```python
from build123d import *

# Parameters (mm, degrees)
BOSS_EXTRUDE1_DEPTH = 6.35
CHAMFER1_SIZE       = 5
CHAMFER1_SIZE_2     = 7.672581673
SKETCH2_R           = 5.25
CUT_EXTRUDE1_DEPTH  = 329.158989668
SKETCH3_R           = 11
CUT_EXTRUDE2_DEPTH  = 329.158989668
SKETCH4_R           = 13
CUT_EXTRUDE3_DEPTH  = 329.158989668


with BuildPart() as part:
    # Sketch1 → Boss-Extrude1 (new body)
    with BuildSketch(Plane.XY):
        with BuildLine():
            Line((-221.187703094, 70), (221.187703094, 70))
            ThreePointArc((221.187703094, 70), (0, -232), (-221.187703094, 70))
        make_face()
    extrude(amount=BOSS_EXTRUDE1_DEPTH)

    # Chamfer1
    # the kernel refuses this chamfer: 7.672581673, 5 mm, written as the material it takes off along each edge
    with BuildSketch(Plane(origin=(-221.187703094, 70, -19.287514673), x_dir=(1, 0, 0), z_dir=(0, 0, 1))) as chamfer1_piece_1:
        with BuildLine():
            Line((CHAMFER1_SIZE, 0), (-2.131765618, -7.131765618))
            ThreePointArc((-2.131765618, -7.131765618), (-1.133115382, -3.68670064), (0, 0))
            Line((0, 0), (CHAMFER1_SIZE, 0))
        make_face()
    extrude(amount=44.925029345, mode=Mode.SUBTRACT)
    with BuildSketch(Plane(origin=(221.187703094, 70, -19.865544851), x_dir=(-1, 0, 0), z_dir=(0, 0, 1))) as chamfer1_piece_2:
        with BuildLine():
            Line((CHAMFER1_SIZE_2, 0), (-1.44240767, 4.732597867))
            ThreePointArc((-1.44240767, 4.732597867), (-0.765078162, 2.465098705), (0, 0))
            Line((0, 0), (CHAMFER1_SIZE_2, 0))
        make_face()
    extrude(amount=46.081089702, mode=Mode.SUBTRACT)

    # Sketch2 → Cut-Extrude1 (cut, through all)
    with BuildSketch(Plane.XY.offset(6.35)):
        with Locations((-190, 0)):
            Circle(SKETCH2_R)
        with Locations((190, 0)):
            Circle(SKETCH2_R)
        with Locations((95, -164.544826719)):
            Circle(SKETCH2_R)
        with Locations((-95, -164.544826719)):
            Circle(SKETCH2_R)
    extrude(amount=-CUT_EXTRUDE1_DEPTH, mode=Mode.SUBTRACT)

    # Sketch3 → Cut-Extrude2 (cut, through all)
    with BuildSketch(Plane.XY.offset(6.35)):
        with Locations((12.5, -30)):
            Circle(SKETCH3_R)
        with Locations((12.5, -55)):
            Circle(SKETCH3_R)
        with Locations((12.5, -80)):
            Circle(SKETCH3_R)
        with Locations((12.5, -105)):
            Circle(SKETCH3_R)
        with Locations((37.5, -30)):
            Circle(SKETCH3_R)
        with Locations((37.5, -55)):
            Circle(SKETCH3_R)
        with Locations((62.5, -30)):
            Circle(SKETCH3_R)
        with Locations((62.5, -55)):
            Circle(SKETCH3_R)
        with Locations((87.5, -30)):
            Circle(SKETCH3_R)
        with Locations((87.5, -55)):
            Circle(SKETCH3_R)
        with Locations((112.5, -30)):
            Circle(SKETCH3_R)
        with Locations((112.5, -55)):
            Circle(SKETCH3_R)
        with Locations((137.5, -30)):
            Circle(SKETCH3_R)
        with Locations((137.5, -55)):
            Circle(SKETCH3_R)
        with Locations((162.5, -30)):
            Circle(SKETCH3_R)
        with Locations((162.5, -55)):
            Circle(SKETCH3_R)
        with Locations((187.5, -30)):
            Circle(SKETCH3_R)
        with Locations((187.5, -55)):
            Circle(SKETCH3_R)
        with Locations((212.5, -30)):
            Circle(SKETCH3_R)
        with Locations((212.5, -55)):
            Circle(SKETCH3_R)
        with Locations((37.5, -80)):
            Circle(SKETCH3_R)
        with Locations((37.5, -105)):
            Circle(SKETCH3_R)
        with Locations((62.5, -80)):
            Circle(SKETCH3_R)
        with Locations((62.5, -105)):
            Circle(SKETCH3_R)
        with Locations((87.5, -80)):
            Circle(SKETCH3_R)
        with Locations((87.5, -105)):
            Circle(SKETCH3_R)
        with Locations((112.5, -80)):
            Circle(SKETCH3_R)
        with Locations((112.5, -105)):
            Circle(SKETCH3_R)
        with Locations((137.5, -80)):
            Circle(SKETCH3_R)
        with Locations((137.5, -105)):
            Circle(SKETCH3_R)
        with Locations((162.5, -80)):
            Circle(SKETCH3_R)
        with Locations((162.5, -105)):
            Circle(SKETCH3_R)
        with Locations((187.5, -80)):
            Circle(SKETCH3_R)
        with Locations((187.5, -105)):
            Circle(SKETCH3_R)
        with Locations((12.5, 30)):
            Circle(SKETCH3_R)
        with Locations((12.5, 55)):
            Circle(SKETCH3_R)
        with Locations((37.5, 55)):
            Circle(SKETCH3_R)
        with Locations((37.5, 30)):
            Circle(SKETCH3_R)
        with Locations((62.5, 55)):
            Circle(SKETCH3_R)
        with Locations((62.5, 30)):
            Circle(SKETCH3_R)
        with Locations((87.5, 55)):
            Circle(SKETCH3_R)
        with Locations((87.5, 30)):
            Circle(SKETCH3_R)
        with Locations((112.5, 55)):
            Circle(SKETCH3_R)
        with Locations((112.5, 30)):
            Circle(SKETCH3_R)
        with Locations((137.5, 55)):
            Circle(SKETCH3_R)
        with Locations((137.5, 30)):
            Circle(SKETCH3_R)
        with Locations((162.5, 55)):
            Circle(SKETCH3_R)
        with Locations((162.5, 30)):
            Circle(SKETCH3_R)
        with Locations((187.5, 55)):
            Circle(SKETCH3_R)
        with Locations((187.5, 30)):
            Circle(SKETCH3_R)
        with Locations((212.5, 55)):
            Circle(SKETCH3_R)
        with Locations((212.5, 30)):
            Circle(SKETCH3_R)
    cut_extrude2 = extrude(amount=-CUT_EXTRUDE2_DEPTH, mode=Mode.SUBTRACT)

    # Mirror2: Cut-Extrude2 across plane
    add(cut_extrude2.mirror(Plane(origin=(0, 0, 0), x_dir=(0, 0, 1), z_dir=(1, 0, 0))), mode=Mode.SUBTRACT)

    # Sketch4 → Cut-Extrude3 (cut, through all)
    with BuildSketch(Plane.XY.offset(6.35)):
        with Locations((-109, -188.793538025)):
            Circle(SKETCH4_R)
        with Locations((109, -188.793538025)):
            Circle(SKETCH4_R)
    extrude(amount=-CUT_EXTRUDE3_DEPTH, mode=Mode.SUBTRACT)


solid = part.part
```
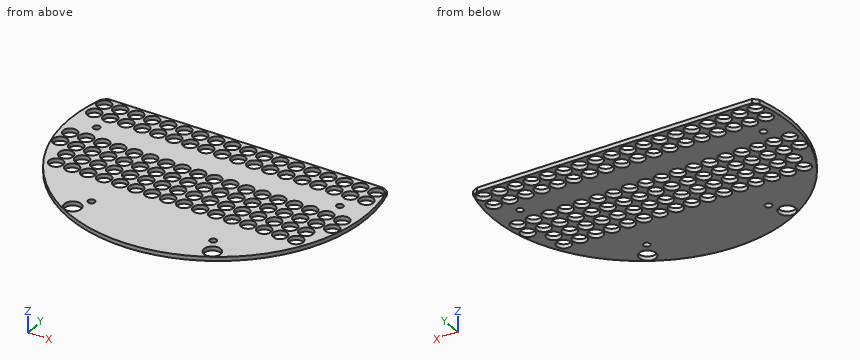
Check sheet for the modelled part. Datum: model origin and axes. Units: mm. Coordinates: 2 decimals unless noted, no trailing zeros. Loops run counter-clockwise (first coordinate to the right, second up) from the corner with the lowest first, then second, coordinate; pieces in that order, holes last.
1) Sectioned sample at A-A (y = 0). Record the boundary of the cut face in (x, z), and give its area (3 significant figures).
2) Gauge pin test, flat ends, axial feed: pin 1 (13 mm diameter, centred on x = -162.5, y = -80, fed in from +Z); pin 2 (3 mm diameter, centred on y = 36.5, z = 1, fed in from +X). Record the tip position at first contact, or that the pin passes through.
3) Sectioned sample at C-C (x = -62.5). Record the boundary of the cut face in (y, z).
4) Material ranges on probe 1 along X at (y, z) = (-184, 1.25); probe 2 along X at (y, z) = (-177, 0.5); probe 3 along X at (y, z) = (10.5, 2.25), recorded low to high.
5) Sectioned sample at D-D (z = 2.75). Count the separate pieces of the cut face and the enclosed holes in it, and give its area (3 significant figures).
6) Sectioned sample at B-B (x = -137.5). Record the boundary of the cut face in (y, z), and give its area (3 significant figures).
Check sheet entries:
1. outline: (-232, 0) - (-195.25, 0) - (-195.25, 6.35) - (-232, 6.35) - close; (-184.75, 0) - (184.75, 0) - (184.75, 6.35) - (-184.75, 6.35) - close; (195.25, 0) - (232, 0) - (232, 6.35) - (195.25, 6.35) - close
1. area: 2,810 mm2
2. pin 1: passes through
2. pin 2: stops at x = 229.34
3. outline: (-223.42, 0) - (-116, 0) - (-116, 6.35) - (-223.42, 6.35) - close; (-94, 0) - (-91, 0) - (-91, 6.35) - (-94, 6.35) - close; (-69, 0) - (-66, 0) - (-66, 6.35) - (-69, 6.35) - close; (-44, 0) - (-41, 0) - (-41, 6.35) - (-44, 6.35) - close; (-19, 0) - (19, 0) - (19, 6.35) - (-19, 6.35) - close; (41, 0) - (44, 0) - (44, 6.35) - (41, 6.35) - close; (66, 0) - (70, 0) - (70, 6.35) - (66, 6.35) - close
4. probe 1: x = -141.31 to -121.08, -96.92 to 96.92, 121.08 to 141.31
4. probe 2: x = -149.98 to -114.47, -103.53 to 103.53, 114.47 to 149.98
4. probe 3: x = -231.76 to 231.76
5. separate pieces: 1
5. enclosed holes: 110
5. area: 75,500 mm2
6. outline: (-186.86, 0) - (-116, 0) - (-116, 6.35) - (-186.86, 6.35) - close; (-94, 0) - (-91, 0) - (-91, 6.35) - (-94, 6.35) - close; (-69, 0) - (-66, 0) - (-66, 6.35) - (-69, 6.35) - close; (-44, 0) - (-41, 0) - (-41, 6.35) - (-44, 6.35) - close; (-19, 0) - (19, 0) - (19, 6.35) - (-19, 6.35) - close; (41, 0) - (44, 0) - (44, 6.35) - (41, 6.35) - close; (66, 0) - (70, 0) - (70, 6.35) - (66, 6.35) - close
6. area: 793 mm2
